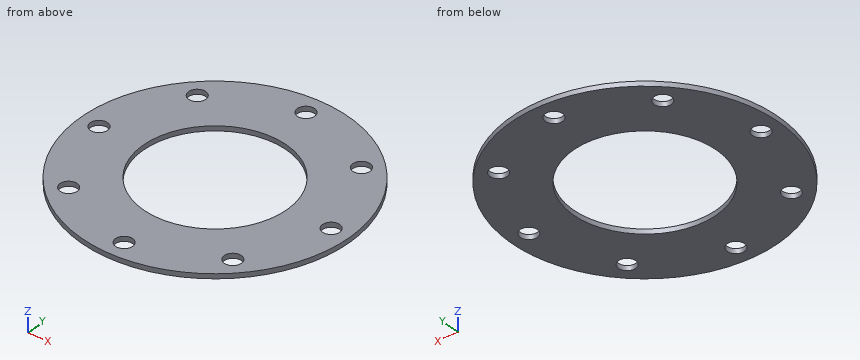
Autodesk Inventor part; units mm, degrees
ref_plane "YZ Plane" through (0, 0, 0) normal (1, 0, 0) x (0, 1, 0)
ref_plane "XZ Plane" through (0, 0, 0) normal (0, 1, 0) x (-1, 0, 0)
ref_plane "XY Plane" through (0, 0, 0) normal (0, 0, 1) x (1, 0, 0)
sketch "Sketch1" plane through (0, 0, 0) normal (0, 0, 1) x (1, 0, 0)
  circle A0 centre (0, 0) radius 75
  circle A1 centre (0, 0) radius 140
  dimension "d22" = 150
  dimension "d23" = 280
extrude "Plate1" add sketch "Sketch1" along normal blind 5
sketch "Sketch5" plane through (0, 0, 5) normal (0, 0, 1) x (1, 0, 0)
  circle A0 centre (0, 120) radius 9
  circle A1 centre (0, 0) radius 120 construction
  dimension "d25" = 240
  dimension "d24" = 18
extrude "Cut1" cut sketch "Sketch5" against normal blind 5
pattern_circular "Circular Pattern1" count 8 over 360 about axis through (0, 0, 0) along (0, 0, 1) of "Cut1"
equation "\"d26\" = Thickness"
equation "\"d2\" = Thickness"
equation "\"BendReliefWidth\" = Thickness"
equation "\"BendReliefDepth\" = 0.5 * Thickness"
equation "\"TransitionRadius\" = BendRadius"
equation "\"JacobiRadiusSize\" = BendRadius"
equation "\"GapSize\" = Thickness"
properties part number "drain flange" material "Stainless Steel"
Here's how the part is built. I have some questions about the finished solid (model axes, mm). Round coordinates to 2 decimals unless told otherwise and drop trailing zeros. Write each loop counter-clockwise with the first axis right and the second up, starting at its lowest first coordinate (ties: lowest second). Pieces come first, ordered by that corner, then holes. Notation, with made-up numbers: M 75.5,-28 L 86.5,-28 A36 cw 86.5,10 Z; hole C 88.5,-4 d3. An arc over 180 degrees is marked long. Answer as CSV lines item,"result". Start each with the question number.
1. Suppose I cut it at B-B on x = 4. Write out the boundary of the cut face in (y, z).
2. Suppose I cut it at D-D on x = -116.5. Write out the boundary of the cut face in (y, z).
3. I need wall thicknesses on probe 1 along Y at (x, z) = (0, 2.5); probe 2 along Y at (x, z) = (89, 2.7); probe 3 along Y at (x, z) = (-5, 2.75). Which ranges of each line are inside material? Lowest first, please.
4. Suppose I cut it at A-A on y = 0. Write out the boundary of the cut face in (x, z).
5. Suppose I cut it at C-C on y = 120. Write out the boundary of the cut face in (x, z), then the cut area to 3 significant figures.
6. I'm going to push flat-ended pins straight in: pin 1 Ø20.5 at (x, y) = (84.85, -84.85) entering from +Z; pin 2 Ø3 at (x, z) = (-45.5, 3) entering from +Y; pin 3 Ø1 at (x, z) = (-37.5, 2.5) entering from +Y; pin 4 Ø2 at (y, z) = (57.5, 1) entering from +X. Where does each tip first touch, or does it pass through?
Check result:
1,outline,"M -139.94,0 L -128.06,0 L -128.06,5 L -139.94,5 Z; M -111.94,0 L -74.89,0 L -74.89,5 L -111.94,5 Z; M 74.89,0 L 111.94,0 L 111.94,5 L 74.89,5 Z; M 128.06,0 L 139.94,0 L 139.94,5 L 128.06,5 Z"
2,outline,"M -77.64,0 L -8.29,0 L -8.29,5 L -77.64,5 Z; M 8.29,0 L 77.64,0 L 77.64,5 L 8.29,5 Z"
3,probe 1,"y = -140 to -129, -111 to -75, 75 to 111, 129 to 140"
3,probe 2,"y = -108.07 to -92.84, -76.87 to 76.87, 92.84 to 108.07"
3,probe 3,"y = -139.91 to -127.48, -112.52 to -74.83, 74.83 to 112.52, 127.48 to 139.91"
4,outline,"M -140,0 L -129,0 L -129,5 L -140,5 Z; M -111,0 L -75,0 L -75,5 L -111,5 Z; M 75,0 L 111,0 L 111,5 L 75,5 Z; M 129,0 L 140,0 L 140,5 L 129,5 Z"
5,outline,"M -72.11,0 L -9,0 L -9,5 L -72.11,5 Z; M 9,0 L 72.11,0 L 72.11,5 L 9,5 Z"
5,area,"631 mm2"
6,pin 1,"stops at z = 5"
6,pin 2,"stops at y = 132.91"
6,pin 3,"stops at y = 135.02"
6,pin 4,"stops at x = 128.09"
